```python
from build123d import *

# Parameters (mm, degrees)
SKETCH2_R          = 27
CUT_EXTRUDE1_DEPTH = 12
SKETCH3_W          = 12
SKETCH3_H          = 6.5


with BuildPart() as part:
    # Sketch1 → Revolve1 (revolve)
    with BuildSketch(Plane.XY, mode=Mode.PRIVATE) as revolve1_sk:
        Polygon((0, 0), (0, 16.2), (9, 16.2), (12, 13.2), (12, 0), align=None)
    revolve(revolve1_sk.sketch.rotate(Axis((12, 0, 0), (-1, 0, 0)), 270), axis=Axis((12, 0, 0), (-1, 0, 0)))

    # Sketch2 → Cut-Extrude1 (cut)
    with BuildSketch(Plane(origin=(0, 0, 0), x_dir=(0, 0, -1), z_dir=(1, 0, 0))):
        Circle(SKETCH2_R)
        Polygon((-13.5, -7.794228634), (0, -15.588457268), (13.5, -7.794228634), (13.5, 7.794228634), (0, 15.588457268), (-13.5, 7.794228634), align=None, mode=Mode.SUBTRACT)
    extrude(amount=CUT_EXTRUDE1_DEPTH, mode=Mode.SUBTRACT)

    # Sketch3 → Cut-Revolve1 (revolve, cut)
    with BuildSketch(Plane.XY, mode=Mode.PRIVATE) as cut_revolve1_sk:
        with Locations((6, 3.25)):
            Rectangle(SKETCH3_W, SKETCH3_H)
    revolve(cut_revolve1_sk.sketch.rotate(Axis((12, 0, 0), (-1, 0, 0)), 270), axis=Axis((12, 0, 0), (-1, 0, 0)), mode=Mode.SUBTRACT)


solid = part.part
```
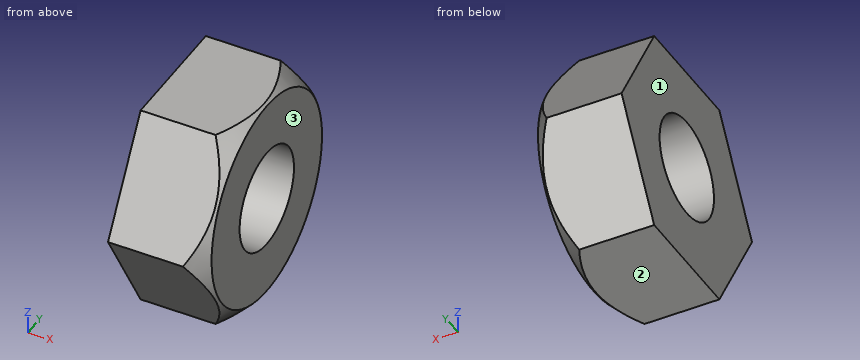
Verification items for the finished model (mm, model axes). Face numbers are marked on the shaded views. Give positions to 0.01 mm unless a question says otherwise; leave off trailing zeros. Write each loop counter-clockwise with the first axis right and the second up, starting at its lowest first coordinate (ties: lowest second). Pieces come first, ordered by that corner, then holes. Notation, with made-up numbers: (18, 9) - (64, 9) arc R10 ccw to (64, 20) - close; hole circle Ø6 at (18.25, 13). An arc over 180 degrees is marked (long way). Put each result on its own line as item: value.
Q1. Section check A-A on y = 0. Record the cut outline in (x, z), and give its area (3 significant figures).
Result:
outline: (0, -13.5) - (11.7, -13.5) - (12, -13.2) - (12, -6.5) - (0, -6.5) - close; (0, 6.5) - (12, 6.5) - (12, 13.2) - (11.7, 13.5) - (0, 13.5) - close
area: 168 mm2
Q2. Depth check by flat-ended pin: P1, Ø2, axis at x = 3.5, z = -2, coming from the -Y side; P2, Ø5, axis at x = 9.5, z = 7, coming from the +Y side. Enter the tip coordinate at first touch or a pass-through.
Result:
P1: y = -15.01
P2: y = 12.99
Q3. Section check B-B on x = 0.5. Record the cut outline in (y, z), and give its area (3 significant figures).
Result:
outline: (-15.59, 0) - (-7.79, -13.5) - (7.79, -13.5) - (15.59, 0) - (7.79, 13.5) - (-7.79, 13.5) - close; hole circle Ø13 at (0, 0)
area: 499 mm2
Q4. Mould release check, pull along X, two halves, no side actions. Record for the marked faces 1, 2 and 3: released by +X, released by -X, zero draft, split by the parting line, or undercut.
Result:
face 1: released by -X
face 2: zero draft
face 3: released by +X
Q5. Section check C-C on x = 11. Record the cut outline in (y, z), and give its area (3 significant figures).
Result:
outline: (-13.89, -2.94) - (-9.49, -10.56) arc R14.2 ccw to (-4.4, -13.5) - (4.4, -13.5) arc R14.2 ccw to (9.49, -10.56) - (13.89, -2.94) arc R14.2 ccw to (13.89, 2.94) - (9.49, 10.56) arc R14.2 ccw to (4.4, 13.5) - (-4.4, 13.5) arc R14.2 ccw to (-9.49, 10.56) - (-13.89, 2.94) arc R14.2 ccw to start; hole circle Ø13 at (0, 0)
area: 476 mm2
Q6. Scan lines: probe 1 along Y at (x, z) = (9, 0); probe 2 along Z at (x, y) = (8.25, -2); probe 3 along Y at (x, z) = (10, 5.75). Record each from-to range of solid material in increasing order. Write a range as from..to.
Result:
probe 1: -15.59..-6.5, 6.5..15.59
probe 2: -13.5..-6.18, 6.18..13.5
probe 3: -12.27..-3.03, 3.03..12.27
